Autodesk Fusion 360 part; units mm, degrees
sketch "Sketch1" plane through (0, 0, 0) normal (0, 0, 1) x (1, 0, 0)
  line L0 (0, 0.05) -> (5, 0.05)
  line L1 (5, 0.05) -> (5, -0.05) construction
  line L2 (5, -0.05) -> (0, -0.05)
  line L3 (0, -0.05) -> (0, 0.05)
  line L4 (5, 0.05) -> (5, 2.5)
  line L5 (5, 2.5) -> (25, 2.5)
  line L6 (25, 2.5) -> (25, 0.1)
  line L7 (25, 0.1) -> (30, 0.1)
  line L8 (30, -0.1) -> (25, -0.1)
  line L9 (25, -0.1) -> (25, -2.5)
  line L10 (25, -2.5) -> (5, -2.5)
  line L11 (5, -2.5) -> (5, -0.05)
  line L12 (30, 0.1) -> (30, 0.2)
  line L13 (19.9, 0.2) -> (19.9, -0.2)
  line L14 (30, -0.4037) -> (30, -0.1)
  line L15 (5.1, 2.4) -> (24.9, 2.4)
  line L16 (24.9, 2.4) -> (24.9, 0.2)
  line L17 (24.9, 0.2) -> (19.9, 0.2)
  line L18 (19.9, 0.2) -> (19.9, -0.2)
  line L19 (19.9, -0.2) -> (24.9, -0.2)
  line L20 (24.9, -0.2) -> (24.9, -2.4)
  line L21 (24.9, -2.4) -> (5.1, -2.4)
  line L22 (5.1, -2.4) -> (5.1, 2.4)
  line L23 (24.9, 0.2) -> (19.9, 0.2)
  line L24 (25, 0.2) -> (24.9, 0.2) construction
  line L25 (19.9, -0.2) -> (24.9, -0.2)
  line L26 (24.9, -0.2) -> (25, -0.6007) construction
  line L27 (30, -0.1) -> (30, -0.2)
  line L28 (30, -0.2) -> (35, -0.2)
  line L29 (35, -0.2) -> (35, 0.2)
  line L30 (35, 0.2) -> (30, 0.2)
  line L31 (30, 0.2) -> (30, 0.1)
  point P0 (19.9, 0)
  point P1 (35, 0)
  dimension "d56" = 0.1
  dimension "d57" = 5
  dimension "d58" = 0.2
  dimension "d59" = 5
  dimension "d60" = 5
  dimension "d64" = 0.1
  dimension "d65" = 0.1
  dimension "d66" = 0.1
  dimension "d67" = 0.1
  dimension "d68" = 0.4
  dimension "d70" = 0.2
  dimension "d71" = 5
  dimension "d72" = 20
  dimension "d73" = 5
  dimension "d74" = 0.1
  dimension "d76" = 5
  dimension "d77" = 0.4
  dimension "d78" = 0.2
  dimension "spacer" = 5
  dimension "d80" = 0.1
  dimension "d81" = 2.5
extrude "Extrude2" add sketch "Sketch1" along normal blind 0.4
equation "d1000 = channelwidth"
equation "d11 = d1000 * 2.2"
equation "d1001 = depth"
equation "mouth_user = 0.1 mm"
equation "mouth_size = d1000 + 0.5 mm"
equation "channelwidth = 0.1 mm"
equation "depth = 0.4 mm"
equation "length = 20 mm"
equation "neckwidth = 0.2 mm"
equation "inputwidth = neckwidth * 2"
equation "outletwidth = inputwidth"
equation "necklength = 5 mm"
equation "d56 = channelwidth"
equation "d57 = spacer"
equation "d58 = neckwidth"
equation "d59 = necklength"
equation "d60 = necklength"
equation "d64 = channelwidth"
equation "d65 = channelwidth"
equation "d66 = channelwidth"
equation "d67 = channelwidth"
equation "d68 = inputwidth"
equation "d70 = inputwidth / 2"
equation "d71 = inputlength"
equation "d72 = length"
equation "d74 = channelwidth"
equation "d76 = inputlength"
equation "d77 = outletwidth"
equation "d78 = outletwidth / 2"
equation "d80 = neckwidth / 2"
equation "d81 = d73 / 2"
equation "inputlength = 5 mm"
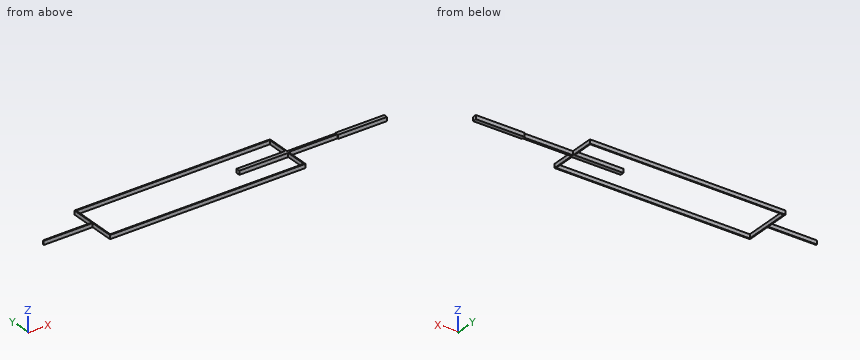
Here's how the part is built. I have some questions about the finished solid (model axes, mm). Give positions to 0.01 mm unless a question says otherwise; leave off trailing zeros. Loops run counter-clockwise (first coordinate to the right, second up) from the corner with the lowest first, then second, coordinate; pieces in that order, holes last. Notation, with made-up numbers: M 34.5,51 L 79.5,51 A10 cw 79.5,62 Z; hole C 78.5,88.5 d2. An arc over 180 degrees is marked long. Use one line per item in the form item = value. Start each with the question number.
Q1. If we section it at B-B (x = 16.5): Write out the boundary of the cut face in (y, z), then the cut area to 3 significant figures.
Q2. I need wall thicknesses on line 1 along X through (y, z) = (0, 0.2); line 2 along Y through (x, z) = (28.5, 0.25). Which ranges of each line are inside material? Lowest first, please.
Q3. If we section it at C-C (x = 21.5): Write out the boundary of the cut face in (y, z).
Q4. If we section it at D-D (z = 0.1): Write out the boundary of the cut face in (x, y), then the cut area to 3 significant figures.
Q5. If we section it at A-A (y = 1.2): Write out the boundary of the cut face in (x, z), then the cut area to 3 significant figures.
Taken from the geometry:
q1.outline = M -2.5,0 L -2.4,0 L -2.4,0.4 L -2.5,0.4 Z; M 2.4,0 L 2.5,0 L 2.5,0.4 L 2.4,0.4 Z
q1.area = 0.0800 mm^2
q2.line_1 = 0 to 5.1, 19.9 to 35
q2.line_2 = -0.1 to 0.1
q3.outline = M -2.5,0 L -2.4,0 L -2.4,0.4 L -2.5,0.4 Z; M -0.2,0 L 0.2,0 L 0.2,0.4 L -0.2,0.4 Z; M 2.4,0 L 2.5,0 L 2.5,0.4 L 2.4,0.4 Z
q4.outline = M 0,-0.05 L 5,-0.05 L 5,-2.5 L 25,-2.5 L 25,-0.1 L 30,-0.1 L 30,-0.2 L 35,-0.2 L 35,0.2 L 30,0.2 L 30,0.1 L 25,0.1 L 25,2.5 L 5,2.5 L 5,0.05 L 0,0.05 Z; hole M 5.1,-2.4 L 24.9,-2.4 L 24.9,-0.2 L 19.9,-0.2 L 19.9,0.2 L 24.9,0.2 L 24.9,2.4 L 5.1,2.4 Z
q4.area = 10.5 mm^2
q5.outline = M 5,0 L 5.1,0 L 5.1,0.4 L 5,0.4 Z; M 24.9,0 L 25,0 L 25,0.4 L 24.9,0.4 Z
q5.area = 0.0800 mm^2
